Autodesk Inventor part; units mm, degrees
ref_plane "YZ Plane" through (0, 0, 0) normal (1, 0, 0) x (0, 1, 0)
ref_plane "XZ Plane" through (0, 0, 0) normal (0, 1, 0) x (-1, 0, 0)
ref_plane "XY Plane" through (0, 0, 0) normal (0, 0, 1) x (1, 0, 0)
sketch "Sketch1" plane through (0, 0, 0) normal (0, 1, 0) x (-1, 0, 0)
  line L0 (990, 495) -> (-990, 495) construction
  line L1 (-990, 495) -> (-990, -495) construction
  line L2 (-990, -495) -> (990, -495) construction
  line L3 (990, -495) -> (990, 495) construction
  line L4 (990, 495) -> (-990, -495) construction
  line L5 (-990, 495) -> (990, -495) construction
  line L6 (890, -395) -> (-890, -395) construction
  line L7 (-890, -395) -> (-890, 395) construction
  line L8 (-890, 395) -> (890, 395) construction
  line L9 (890, 395) -> (890, -395) construction
  circle A0 centre (890, -395) radius 25
  circle A1 centre (-890, -395) radius 25
  circle A2 centre (890, 395) radius 25
  circle A3 centre (-890, 395) radius 25
  point P0 (0, 0)
  dimension "d0" = 1980
  dimension "d1" = 990
  dimension "d2" = 100
  dimension "d3" = 50
extrude "Extrusion1" add sketch "Sketch1" along normal blind 150
sketch "Sketch2" plane through (0, 150, 0) normal (0, 1, 0) x (-1, 0, 0)
  line L0 (990, -495) -> (990, 495)
  line L1 (-990, -495) -> (990, -495)
  line L2 (-990, 495) -> (-990, -495)
  line L3 (990, 495) -> (-990, 495)
  point P0 (0, 0)
extrude "Extrusion2" add sketch "Sketch2" along normal blind 150
sketch "Sketch3" plane through (0, 300, 0) normal (0, 1, 0) x (1, 0, 0)
  line L0 (-990, 495) -> (990, 495)
  line L1 (990, 495) -> (990, 395)
  line L2 (990, 395) -> (-990, 395)
  line L3 (-990, 395) -> (-990, 495)
  line L4 (990, 395) -> (890, 395)
  line L5 (890, 395) -> (890, -255)
  line L6 (890, -255) -> (990, -255)
  line L7 (990, -255) -> (990, 395)
  line L8 (-990, 395) -> (-890, 395)
  line L9 (-890, 395) -> (-890, -255)
  line L10 (-890, -255) -> (-990, -255)
  line L11 (-990, -255) -> (-990, 395)
  line L12 (990, -495) -> (990, 495)
  point P0 (0, 0)
  dimension "d8" = 100
  dimension "d10" = 650
extrude "Extrusion3" add sketch "Sketch3" along normal blind 250
properties part number "Divano"
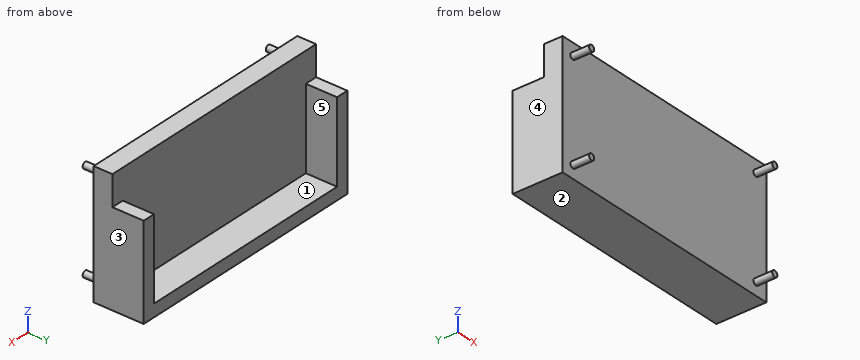
The listing builds one solid part. Answer for the finished solid, in the listing's coordinates (mm). Face numbers are marked on the shaded views. A direction names the side the tool comes from. Coordinates: 2 decimals unless noted, no trailing zeros. Write each loop counter-clockwise with the first axis right and the second up, starting at its lowest first coordinate (ties: lowest second). Pieces come first, ordered by that corner, then holes. Notation, with made-up numbers: (84, -19.75) - (126, -19.75) arc R21 ccw to (126, 1.25) - close; hole circle Ø2 at (8.25, 48.5). An arc over 180 degrees is marked (long way). Return JSON: item names as keys, results as strings. Group by question number.
1. A cutting plane is placed at A-A, the plane z = -49.5. Determine the outline of the cut face in (x, y), plus the area to 3 significant figures.
2. A cutting plane is placed at B-B, the plane y = 482. Determine the outline of the cut face in (x, z), plus the area to 3 significant figures.
3. Which of the six approach directions +Z, -Z, +X, -X, +Y, -Y give full straight-line access (tool end or side, diameter ignored) to the marked faces 1 and 2?
4. A cutting plane is placed at C-C, the plane y = 40.5. Determine the outline of the cut face in (x, z).
5. Straight lines are drawn through the part: L1, parallel to X at y = 476, z = -72; L2, parallel to Z at x = -826.5, y = 520; L3, parallel to Y at x = 650.5, z = 210.5. For each, find the intervals that lie inside material, in ascending order.
6. Determine the mould class of the marked faces 3, 4 and 5 for opening direction X: released by +X, released by -X, zero draft, split by the parting line, or undercut.
7. Given pin 1 (4 mm diameter, centred on x = 343.5, z = 102, fed in from +Y); pin 2 (1 mm diameter, centred on x = 449.5, z = 168, fed in from -Y); pin 3 (10 mm diameter, centred on x = -44.5, y = 415, fed in from +Z), each flat-ended and moving along its own axis, determine where each tip first touches the part or whether it passes through.
8. A cutting plane is placed at D-D, the plane x = 339. Determine the outline of the cut face in (y, z).
Ans:
{
 "1": {"outline": "(-990, 150) - (990, 150) - (990, 550) - (890, 550) - (890, 300) - (-890, 300) - (-890, 550) - (-990, 550) - close", "area": "347,000 mm²"},
 "2": {"outline": "(-990, -495) - (990, -495) - (990, 255) - (890, 255) - (890, -395) - (-890, -395) - (-890, 255) - (-990, 255) - close", "area": "328,000 mm²"},
 "3": {"face 1": "+Z, +Y", "face 2": "-Z, +X, -X, +Y, -Y"},
 "4": {"outline": "circle Ø50 at (-890, -395); circle Ø50 at (-890, 395); circle Ø50 at (890, -395); circle Ø50 at (890, 395)"},
 "5": {"L1": "-990 to -890, 890 to 990", "L2": "-495 to -395", "L3": "150 to 300"},
 "6": {"face 3": "released by +X", "face 4": "released by -X", "face 5": "undercut"},
 "7": {"pin 1": "y = 300", "pin 2": "y = 150", "pin 3": "z = -395"},
 "8": {"outline": "(150, -495) - (550, -495) - (550, -395) - (300, -395) - (300, 495) - (150, 495) - close"}
}
